Answer from the drawing. Dimensions are ordinates in mm from the lowest x, y and z of the part. A direction names the side the tool comes from. Round coordinates to 2 decimals unless told otherwise and drop trailing zeros. Loops run counter-clockwise (first coordinate to the right, second up) from the corner with the lowest first, then second, coordinate; pieces in that order, holes last. Notation, with made-up numbers: (-26, 29) -> (-17, 29) arc R17 ccw to (-17, 36) -> close; hole circle Ø8 at (11.5, 43). An arc over 180 degrees is marked (long way). One line per question, with ' | ' between items.
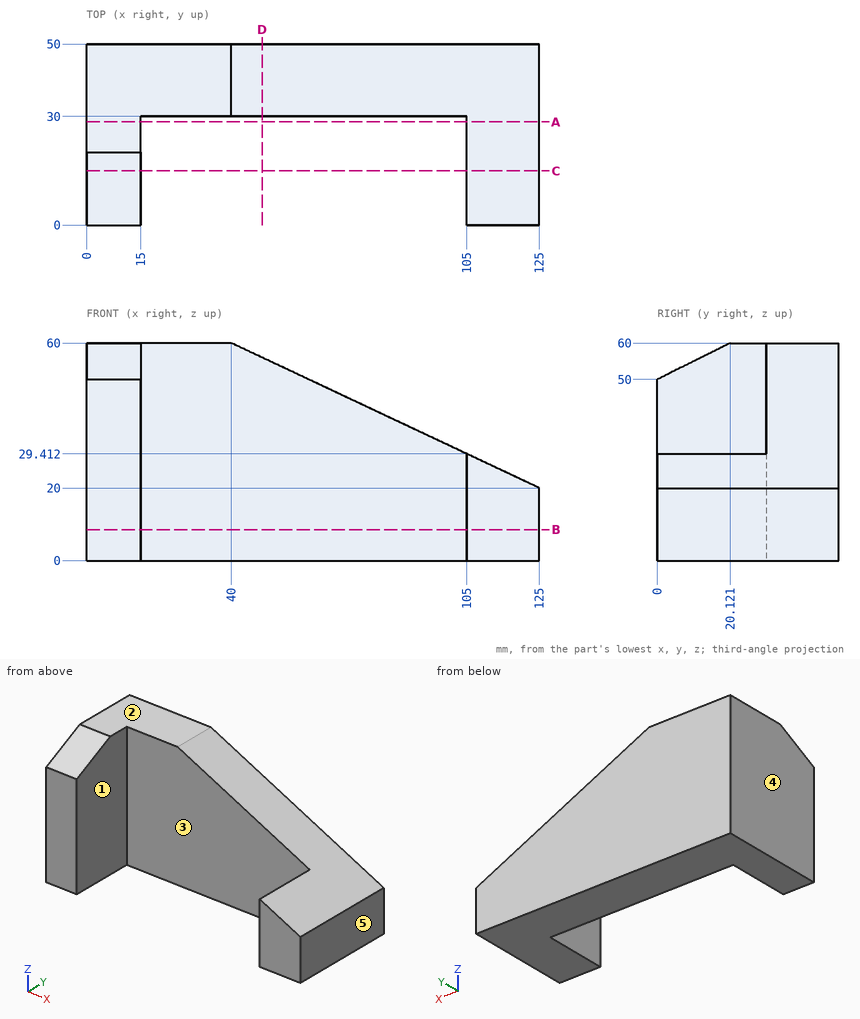
Q1. A cutting plane is placed at C-C on y = 15. Give the vertices of the cut face in (x, z) (1 decimal).
Numbers:
outline: (0, 0) -> (15, 0) -> (15, 57.5) -> (0, 57.5) -> close; (105, 0) -> (125, 0) -> (125, 20) -> (105, 29.4) -> close
Q2. A cutting plane is placed at D-D on x = 48.5. Give the vertices of the cut face in (y, z), plus the area to 3 significant figures.
Numbers:
outline: (30, 0) -> (50, 0) -> (50, 56) -> (30, 56) -> close | area: 1,120 mm^2
Q3. For the marked faces 1 and 2, determine the directions among +Z, -Z, +X, -X, +Y, -Y from which every point of the face is accessible in a straight line to the end or side of a thin tool.
Numbers:
face 1: +Z, -Z, -Y | face 2: +Z, +X, -X, +Y, -Y
Q4. Find the intervals of material crossed by line 1 (X direction, y = 8, z = 11.5); line 2 (Y direction, x = 61, z = 14.5); line 3 (X direction, y = 3, z = 42), in increasing order. Write a range as from..to.
Numbers:
line 1: 0..15, 105..125 | line 2: 30..50 | line 3: 0..15
Q5. A cutting plane is placed at B-B on z = 8.5. Give the vertices of the cut face in (x, y), plus the area to 3 significant figures.
Numbers:
outline: (0, 0) -> (15, 0) -> (15, 30) -> (105, 30) -> (105, 0) -> (125, 0) -> (125, 50) -> (0, 50) -> close | area: 3,550 mm^2
Q6. For a pull along X with two mould halves and no side action, classify the marked faces 3, 4 and 5 as pulls with the +X half, pulls with the -X half, needs draft (parallel to the pull), parting line crosses it, or undercut.
Numbers:
face 3: undercut | face 4: pulls with the -X half | face 5: pulls with the +X half
Q7. A cutting plane is placed at A-A on y = 28.5. Give the vertices of the cut face in (x, z), plus the area to 3 significant figures.
Numbers:
outline: (0, 0) -> (15, 0) -> (15, 60) -> (0, 60) -> close; (105, 0) -> (125, 0) -> (125, 20) -> (105, 29.41) -> close | area: 1,390 mm^2
Q8. Given pin 1 Ø24 at (y, z) = (18.5, 32.5) entering from +X; pin 2 Ø3 at (y, z) = (28, 47) entering from +X; pin 3 Ø2 at (y, z) = (15.5, 28.5) entering from +X, each flat-ended and moving along its own axis, determine where each tip first touches the part or whether it passes through.
Numbers:
pin 1: x = 123.94 | pin 2: x = 15 | pin 3: x = 109.06
